Design review of the part built by this model. Coordinates are the model's own, in mm. Give positions to 0.01 mm unless a question says otherwise; leave off trailing zeros. Loops run counter-clockwise (first coordinate to the right, second up) from the corner with the lowest first, then second, coordinate; pieces in that order, holes last. Notation, with made-up numbers: M 63.25,21.5 L 67.25,21.5 A32 ccw 67.25,52.5 Z; hole C 88.5,89.25 d5. An arc over 180 degrees is marked long. Use a Markdown table: item, result. Add a question column.
(1) Add section B-B, the plane x = 43. Give the boundary of the cut face in (y, z), then the cut area to 3 significant figures.
(2) For probe 1 along X at (y, z) = (8, 1.5); probe 2 along X at (y, z) = (7, -2.75); probe 3 along Y at (x, z) = (178.5, 9.75), list the stretches that pass through material, from the lowest coordinate up.
(3) Insertion check: pin 1 Ø3.5 at (x, z) = (89.5, -0.5) entering from +Y; pin 2 Ø3 at (x, z) = (107.5, 11) entering from +Y; pin 3 Ø3 at (y, z) = (7.5, -1) entering from +X; pin 4 Ø1.9 at (x, y) = (75.5, 7) entering from +Z. Each pin has a flat end and moves straight along its axis. Give the tip position at first contact, or say it passes through.
(4) Add section A-A, the plane z = 6. Give the boundary of the cut face in (x, y), then the cut area to 3 significant figures.
(5) Draft analysis for pull direction X (two halves, no side actions). For faces 1 (the face through (80, 2, 13.274)), 2 (the face through (207.078, 2, 3)), 3 (the face through (81.995, 4.976, -1.656)), 4 (the face through (-42.922, 2, 3)), state which applies: pulls with the +X half, pulls with the -X half, needs draft (parallel to the pull), parting line crosses it, or undercut.
```python
from build123d import *

# Parameters (mm, degrees)
SKETCH1_W           = 250
SKETCH1_H           = 20
BOSS_EXTRUDE1_DEPTH = 5
SKETCH2_W           = 20
SKETCH2_H           = 10
BOSS_EXTRUDE2_DEPTH = 3.75
SKETCH3_R           = 3.775
CUT_EXTRUDE1_DEPTH  = 10
SKETCH4_R           = 1.5
CUT_EXTRUDE2_DEPTH  = 4


with BuildPart() as part:
    # Sketch1 → Boss-Extrude1 (new body)
    with BuildSketch(Plane(origin=(0, 0, 0), x_dir=(1, 0, 0), z_dir=(0, 1, 0))):
        with Locations((82.077816098, -3.273623345)):
            Rectangle(SKETCH1_W, SKETCH1_H)
    extrude(amount=BOSS_EXTRUDE1_DEPTH)

    # Sketch2 → Boss-Extrude2 (add)
    with BuildSketch(Plane(origin=(0, 5, 0), x_dir=(1, 0, 0), z_dir=(0, 1, 0))):
        with Locations((82.077816098, 1.726376655)):
            Rectangle(SKETCH2_W, SKETCH2_H)
    extrude(amount=BOSS_EXTRUDE2_DEPTH)

    # Sketch3 → Cut-Extrude1 (cut)
    with BuildSketch(Plane.XY.offset(3.273623345)):
        with Locations((82.077816098, 8.75)):
            Circle(SKETCH3_R)
    extrude(amount=-CUT_EXTRUDE1_DEPTH, mode=Mode.SUBTRACT)

    # Sketch4 → Cut-Extrude2 (cut)
    with BuildSketch(Plane(origin=(0, 8.75, 0), x_dir=(1, 0, 0), z_dir=(0, 1, 0))):
        with Locations(Location((89.077816098, -0.273623345, 0), (0, 0, 270))):
            Circle(SKETCH4_R)
        with Locations(Location((75.077816098, 3.726376655, 0), (0, 0, 270))):
            Circle(SKETCH4_R)
    extrude(amount=-CUT_EXTRUDE2_DEPTH, mode=Mode.SUBTRACT)


solid = part.part
```
Established:
| question | item | result |
|---|---|---|
| 1 | outline | M 0,-6.73 L 5,-6.73 L 5,13.27 L 0,13.27 Z |
| 1 | area | 100 mm^2 |
| 2 | probe 1 | 72.08 to 78.38, 85.78 to 88.21, 89.94 to 92.08 |
| 2 | probe 2 | 72.08 to 73.94, 76.22 to 78.73, 85.42 to 92.08 |
| 2 | probe 3 | 0 to 5 |
| 3 | pin 1 | y = 8.75 |
| 3 | pin 2 | y = 5 |
| 3 | pin 3 | x = 92.08 |
| 3 | pin 4 | z = 3.27 |
| 4 | outline | M -42.92,0 L 207.08,0 L 207.08,5 L -42.92,5 Z |
| 4 | area | 1,250 mm^2 |
| 5 | face 1 | needs draft |
| 5 | face 2 | pulls with the +X half |
| 5 | face 3 | undercut |
| 5 | face 4 | pulls with the -X half |
